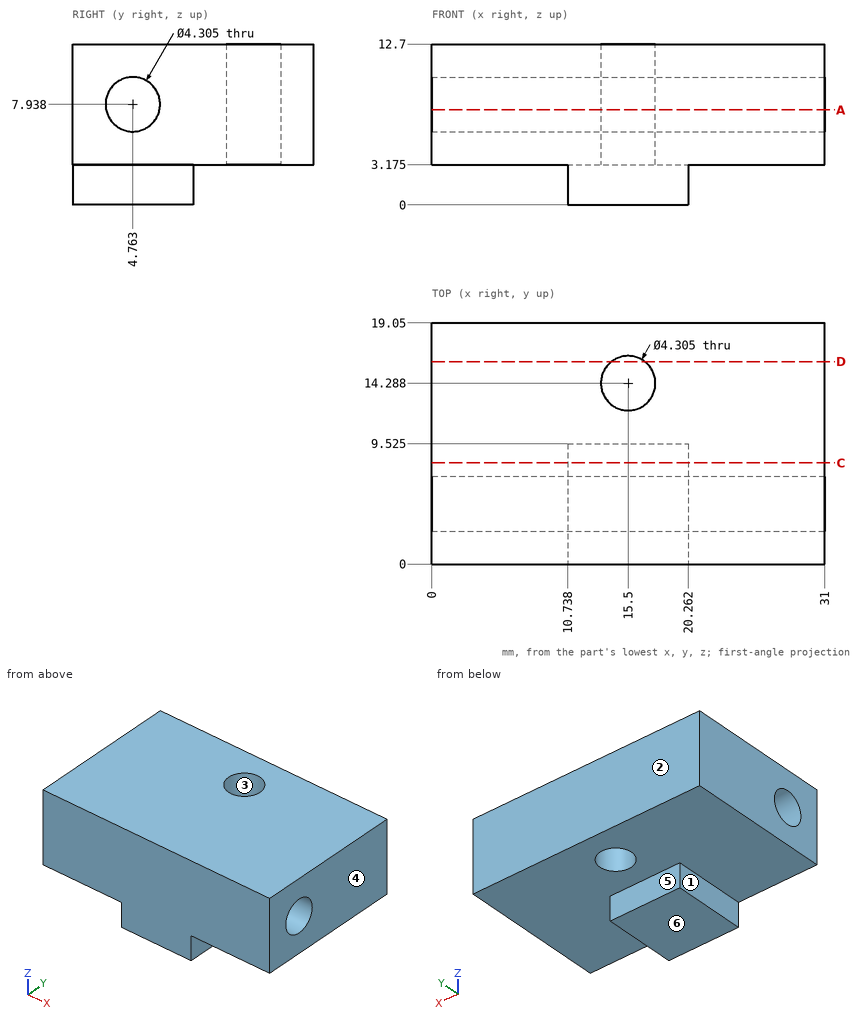
For this review, use the dimensioned drawing (mm, ordinates from the lowest corner) and the shaded views. A direction names the side the tool comes from. Round coordinates to 2 decimals unless told otherwise and drop trailing zeros. Loops run counter-clockwise (first coordinate to the right, second up) from the corner with the lowest first, then second, coordinate; pieces in that order, holes last. Notation, with made-up numbers: M 66.5,29 L 73.5,29 A9 cw 73.5,40 Z; hole C -6.5,-39 d11. An arc over 180 degrees is marked long. Answer as a JSON object with one key per item and string values.
(1) To check wall thickness, follow line 1 along Z through (x, y) = (21, 10.25) (1 decimal); line 2 along Y through (x, z) = (19, 8.25); line 3 along Z through (x, y) = (9, 4.5) (1 decimal). State the ranges of each line that lie inside material, in increasing order.
Resolved:
{"line 1": "3.2 to 12.7", "line 2": "0 to 2.63, 6.89 to 19.05", "line 3": "3.2 to 5.8, 10.1 to 12.7"}
(2) Take a section at D-D on y = 16. Give the boundary of the cut face in (x, z) (1 decimal).
Resolved:
{"outline": "M 0,3.2 L 14.2,3.2 L 14.2,12.7 L 0,12.7 Z; M 16.8,3.2 L 31,3.2 L 31,12.7 L 16.8,12.7 Z"}
(3) Draft analysis for pull direction X (two halves, no side actions). For the marked faces 1, 2, 3 and 4, state which applies: released by +X, released by -X, zero draft, split by the parting line, or undercut.
Resolved:
{"face 1": "released by -X", "face 2": "zero draft", "face 3": "undercut", "face 4": "released by +X"}
(4) Take a section at C-C on y = 8. Give the boundary of the cut face in (x, z) (1 decimal).
Resolved:
{"outline": "M 0,3.2 L 10.7,3.2 L 10.7,0 L 20.3,0 L 20.3,3.2 L 31,3.2 L 31,12.7 L 0,12.7 Z"}
(5) Tool access review of the marked faces 5 and 6: name each direction out of +Z, -Z, +X, -X, +Y, -Y from which nothing blocks a thin tool from reaching the whole face with its end or side.
Resolved:
{"face 5": "-Z, +X, -X, +Y", "face 6": "-Z, +X, -X, +Y, -Y"}
(6) Take a section at A-A on z = 7.5. Count the separate pieces of the cut face and the enclosed holes in it, and give its area (3 significant figures).
Resolved:
{"separate pieces": "2", "enclosed holes": "1", "area": "445 mm²"}
(7) Clearance check with flat-ended pins moving along their axes: P1, Ø3.5, axis at y = 4.5, z = 1.5, coming from the +X side; P2, Ø1.6, axis at x = 17, z = 1.5, coming from the +Y side (1 decimal); P3, Ø10, axis at x = 27, y = 4.5, coming from the -Z side (1 decimal); P4, Ø2.5, axis at y = 7, z = 1.5, coming from the -X side. State where each tip first meets the part, or that it passes through.
Resolved:
{"P1": "x = 31", "P2": "y = 9.5", "P3": "z = 3.2", "P4": "x = 10.74"}
